Job drawing, mm, ordinate dimensions from the low corner. One solid piece. A direction names the side the tool comes from. Give positions to 0.01 mm unless a question says otherwise; leave off trailing zeros. Write each loop counter-clockwise with the first axis right and the second up, starting at its lowest first coordinate (ties: lowest second). Pieces come first, ordered by that corner, then holes. Notation, with made-up numbers: M -20.5,58 L 7.5,58 A13 cw 7.5,82 Z; hole C -21.5,61.25 d11. An arc over 180 degrees is marked long. Use a Markdown table: item, result.
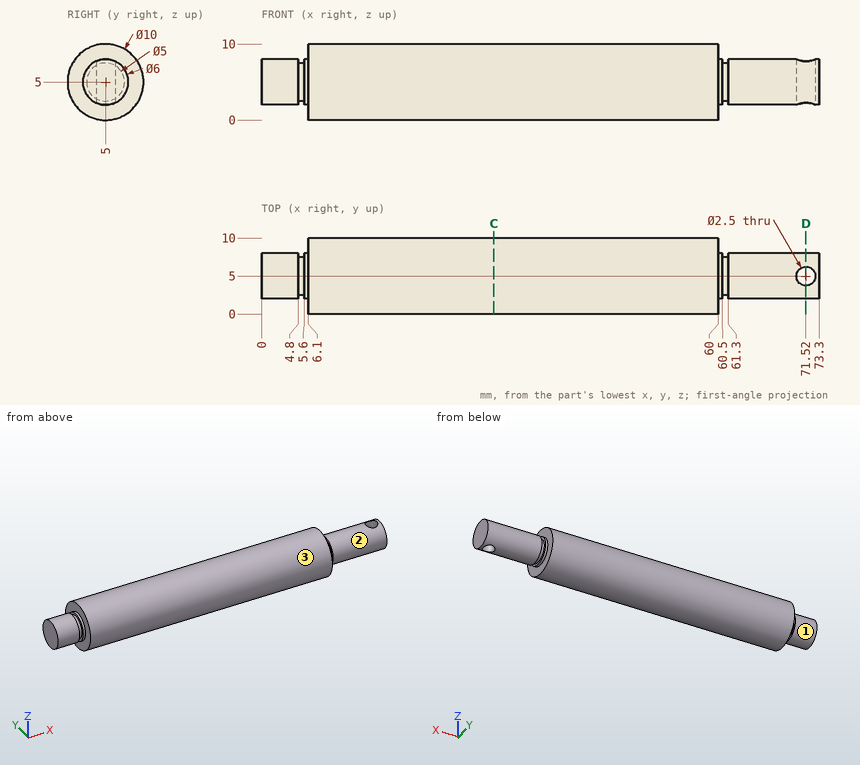
1. Cut at C-C, the plane x = 30.5. Give the cut face in (y, z), then the cut area to 3 significant figures.
Findings below:
| item | result |
|---|---|
| outline | C 5,5 d10 |
| area | 78.5 mm2 |
2. Drop flat-ended pins along their axis: P1, Ø5, axis at x = 50.5, y = 1.5, coming from the +Z side; P2, Ø3, axis at x = 24, z = 6.5, coming from the +Y side; P3, Ø3, axis at x = 71.52, y = 5, coming from the -Z side; P4, Ø6, axis at x = 22.5, y = 1.5, coming from the +Z side. Give the stop position or say it passes through.
Findings below:
| item | result |
|---|---|
| P1 | z = 9.9 |
| P2 | y = 10 |
| P3 | z = 2 |
| P4 | z = 9.97 |
3. Tool access for the marked faces 1, 2 and 3: list every direction of +Z, -Z, +X, -X, +Y, -Y with a clear straight run to the whole face (end or side of a thin tool).
Findings below:
| item | result |
|---|---|
| face 1 | -X |
| face 2 | +X |
| face 3 | +X, -X |
4. Cut at D-D, the plane x = 71.52. Give the cut face in (y, z).
Findings below:
| item | result |
|---|---|
| outline | M 3.75,2.27 L 3.75,7.73 A3 ccw Z; M 6.25,2.27 A3 ccw 6.25,7.73 Z |
5. Drill centre lines: L1, parallel to Y at x = 71.52, z = 5; L2, parallel to X at y = 5, z = 6.5; L3, parallel to X at y = 5, z = 9.25. Where is each one in solid material? Low to high.
Findings below:
| item | result |
|---|---|
| L1 | 2 to 3.75, 6.25 to 8 |
| L2 | 0 to 70.27, 72.77 to 73.3 |
| L3 | 6.1 to 60 |
